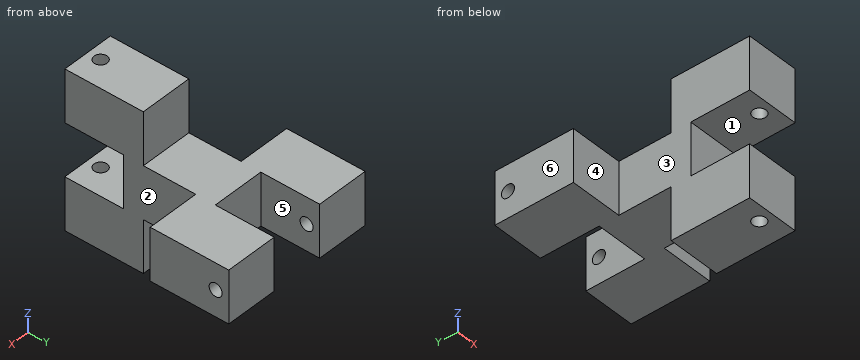
from build123d import *

# Parameters (mm, degrees)
F0_W      = 25.4
F0_H      = 25.4
F1_DEPTH  = 25.4
F3_DEPTH  = 25.4
F4_W      = 76.2
F4_H      = 76.2
F5_DEPTH  = 38.1
F6_W      = 25.4
F6_H      = 38.1
F7_DEPTH  = 101.6
F8_W      = 28.575
F8_H      = 25.4
F9_DEPTH  = 25.4
F10_R     = 3.175
F11_DEPTH = 101.6
F12_R     = 3.175
F13_DEPTH = 127


with BuildPart() as f1:
    # F0 (on Front) → F1 (new body)
    with BuildSketch(Plane.XZ):
        with Locations((-12.7, 12.7)):
            Rectangle(F0_W, F0_H)
    extrude(amount=F1_DEPTH)

    # F2 (on Top) → F3 (join)
    with BuildSketch(Plane.XY):
        Polygon((25.4, 0), (25.4, 38.1), (0, 38.1), (0, 9.525), (-25.4, 9.525), (-25.4, 38.1), (-50.8, 38.1), (-50.8, 0), align=None)
    extrude(amount=F3_DEPTH)

    # F4 (on face) → F5 (join)
    with BuildSketch(Plane.XZ.offset(25.4)):
        with Locations((-12.7, 12.7)):
            Rectangle(F4_W, F4_H)
    extrude(amount=F5_DEPTH)

    # F6 (on face) → F7 (cut)
    with BuildSketch(Plane.XY.offset(50.8)):
        with Locations((12.7, -44.45)):
            Rectangle(F6_W, F6_H)
        with Locations((-38.1, -44.45)):
            Rectangle(F6_W, F6_H)
    extrude(amount=-F7_DEPTH, mode=Mode.SUBTRACT)

    # F8 (on face) → F9 (cut)
    with BuildSketch(Plane.YZ):
        with Locations((-49.2125, 12.7)):
            Rectangle(F8_W, F8_H)
    extrude(amount=-F9_DEPTH, mode=Mode.SUBTRACT)

    # F10 (on face) → F11 (cut)
    with BuildSketch(Plane.XY.offset(50.8)):
        with Locations((-12.7, -57.15)):
            Circle(F10_R)
    extrude(amount=-F11_DEPTH, mode=Mode.SUBTRACT)

    # F12 (on face) → F13 (cut)
    with BuildSketch(Plane.YZ.offset(25.4)):
        with Locations((31.75, 12.7)):
            Circle(F12_R)
    extrude(amount=-F13_DEPTH, mode=Mode.SUBTRACT)


solid = f1.part
Build history of the part. All positions in model axes, mm. Face numbers are marked on the shaded views. A direction names the side the tool comes from. Coordinates: 2 decimals unless noted, no trailing zeros. Order: outer loops, then holes, each group sorted by start corner. A loop starts at its lowest first (then second) coordinate and runs counter-clockwise, first axis right, second up. Notation, with made-up numbers: (23, 6) -> (41, 6) arc R18 cw to (41, 15) -> close; hole circle Ø3 at (59.5, 8.5). An arc over 180 degrees is marked (long way). One line per item, written item: value.
(1) Slice it at C-C, the plane z = 12.7. List the corners of the cut face in (x, y) (3 decimals), plus the area to 3 significant figures.
Checked values:
outline: (-50.8, 0) -> (-25.4, 0) -> (-25.4, -34.925) -> (0, -34.925) -> (0, 0) -> (25.4, 0) -> (25.4, 28.575) -> (0, 28.575) -> (0, 9.525) -> (-25.4, 9.525) -> (-25.4, 28.575) -> (-50.8, 28.575) -> close; (-50.8, 34.925) -> (-25.4, 34.925) -> (-25.4, 38.1) -> (-50.8, 38.1) -> close; (0, 34.925) -> (25.4, 34.925) -> (25.4, 38.1) -> (0, 38.1) -> close
area: 2,740 mm2
(2) Tool access for the marked faces 1, 2 and 3: list every direction of +Z, -Z, +X, -X, +Y, -Y with a clear straight run to the whole face (end or side of a thin tool).
Checked values:
face 1: +X, -X, -Y
face 2: +Z, -Z, +X, -Y
face 3: +Z, -Z, -X, -Y
(3) Slice it at A-A, the plane x = -12.7. List the corners of the cut face in (y, z) (3 decimals), plus the area to 3 significant figures.
Checked values:
outline: (-63.5, -25.4) -> (-60.325, -25.4) -> (-60.325, 0) -> (-63.5, 0) -> close; (-63.5, 25.4) -> (-60.325, 25.4) -> (-60.325, 50.8) -> (-63.5, 50.8) -> close; (-53.975, -25.4) -> (-25.4, -25.4) -> (-25.4, 0) -> (9.525, 0) -> (9.525, 25.4) -> (-25.4, 25.4) -> (-25.4, 50.8) -> (-53.975, 50.8) -> (-53.975, 25.4) -> (-34.925, 25.4) -> (-34.925, 0) -> (-53.975, 0) -> close
area: 2,740 mm2
(4) Slice it at B-B, the plane y = -49. List the corners of the cut face in (x, z), plus the area to 3 significant figures.
Checked values:
outline: (-25.4, -25.4) -> (0, -25.4) -> (0, 0) -> (-25.4, 0) -> close; (-25.4, 25.4) -> (0, 25.4) -> (0, 50.8) -> (-25.4, 50.8) -> close
area: 1,290 mm2
(5) Slice it at D-D, the plane x = -33.5. List the corners of the cut face in (y, z) (3 decimals), plus the area to 3 significant figures.
Checked values:
outline: (0, 0) -> (38.1, 0) -> (38.1, 25.4) -> (0, 25.4) -> close; hole circle Ø6.35 at (31.75, 12.7)
area: 936 mm2
(6) Drop flat-ended pins along their axis: pin 1 Ø1.5 at (x, y) = (5, 7.5) entering from -Z; pin 2 Ø12.5 at (x, z) = (-15, 42.5) entering from +Y; pin 3 Ø12 at (x, z) = (10.5, 6) entering from -Y. Give the stop position or say it passes through.
Checked values:
pin 1: z = 0
pin 2: y = -25.4
pin 3: y = 0
(7) Mould opens along X. For the marked faces 4, 5 and 6 say: pulls with the +X half, pulls with the -X half, needs draft (parallel to the pull), parting line crosses it, or undercut.
Checked values:
face 4: needs draft
face 5: undercut
face 6: pulls with the -X half
(8) Probe line 1 (X direction, y = -57, z = -17); line 2 (X direction, y = 19, z = 13); line 3 (Z direction, x = 18.75, y = 31.75) (3 decimals). List the from-to ranges inside material, lowest first. Write a range as [from, to].
Checked values:
line 1: [-25.4, -15.87], [-9.53, 0]
line 2: [-50.8, -25.4], [0, 25.4]
line 3: [0, 9.525], [15.875, 25.4]
